Read the model definition and answer for the solid it produces. Units are mm, in the model's axes. A direction names the side the tool comes from. Give positions to 0.01 mm unless a question says otherwise; leave off trailing zeros. Order: outer loops, then holes, each group sorted by start corner. A loop starts at its lowest first (then second) coordinate and runs counter-clockwise, first axis right, second up.
Item 1: The mould has two halves that part along X. Classify faces 3 (the face through (0, 0.864, 0)), 4 (the face through (-15.875, 3, 0)), 5 (the face through (0, 5.423, 0)): +X half, -X half, draft (parallel to the pull), parting line (faces both ways), or undercut.
Item 2: Which of the six approach directions +Z, -Z, +X, -X, +Y, -Y give full straight-line access (tool end or side, diameter ignored) to faces 1 (the face through (-4, 0, -13)), 2 (the face through (11.968, 0.4, -0.1))?
Item 3: A cutting plane is placed at A-A (x = 0). Write down the section's boundary in (y, z) (3 decimals), plus the area to 3 significant figures.
Item 4: Given pin 1 Ø8 at (x, z) = (-10, -5) entering from -Y; pin 2 Ø16 at (x, z) = (0, 0) entering from -Y, each flat-ended and moving along its own axis, determine where each tip first touches the part or whether it passes through.
Item 5: Find the intervals of material crossed by line 1 along Z through (x, y) = (0, 0.45) (3 decimals); line 2 along Y through (x, z) = (6, 1.75); line 3 along X through (y, z) = (0.3, 0) (3 decimals), in increasing order.
Item 6: A cutting plane is placed at B-B (z = 0). Write down the section's boundary in (x, y) (3 decimals).
from build123d import *

# Parameters (mm, degrees)
SKETCH3_W           = 31.75
SKETCH3_H           = 29.21
BOSS_EXTRUDE2_DEPTH = 5.4229
CUT_EXTRUDE1_DEPTH  = 0.8636


with BuildPart() as part:
    # Sketch3 → Boss-Extrude2 (new body)
    with BuildSketch(Plane(origin=(0, 0, 0), x_dir=(1, 0, 0), z_dir=(0, 1, 0))):
        Rectangle(SKETCH3_W, SKETCH3_H)
    extrude(amount=BOSS_EXTRUDE2_DEPTH)

    # Sketch1 → Cut-Extrude1 (cut)
    with BuildSketch(Plane(origin=(0, 0, 0), x_dir=(1, 0, 0), z_dir=(0, 1, 0))):
        with BuildLine():
            Line((11.967686493, 5.588), (11.967686493, -5.588))
            ThreePointArc((11.967686493, -5.588), (-13.208, 0), (11.967686493, 5.588))
        make_face()
    extrude(amount=CUT_EXTRUDE1_DEPTH, mode=Mode.SUBTRACT)


solid = part.part
Response values:
1. face 3: undercut
1. face 4: -X half
1. face 5: draft
2. face 1: +Z, -Z, +X, -X, -Y
2. face 2: -Y
3. outline: (0, -14.605) - (5.423, -14.605) - (5.423, 14.605) - (0, 14.605) - (0, 13.208) - (0.864, 13.208) - (0.864, -13.208) - (0, -13.208) - close
3. area: 136 mm2
4. pin 1: stops at y = 0
4. pin 2: stops at y = 0.86
5. line 1: z = -14.605 to -13.208, 13.208 to 14.605
5. line 2: y = 0.86 to 5.42
5. line 3: x = -15.875 to -13.208, 11.968 to 15.875
6. outline: (-15.875, 0) - (-13.208, 0) - (-13.208, 0.864) - (11.968, 0.864) - (11.968, 0) - (15.875, 0) - (15.875, 5.423) - (-15.875, 5.423) - close
